Check sheet for the modelled part. Datum: model origin and axes. Units: mm. Face numbers are marked on the shaded views. A direction names the side the tool comes from. Give positions to 0.01 mm unless a question says otherwise; leave off trailing zeros. Order: outer loops, then holes, each group sorted by start corner. A loop starts at its lowest first (then second) coordinate and runs counter-clockwise, first axis right, second up.
from build123d import *

# Parameters (mm, degrees)
ESQUISSE1_R             = 6
BOSS_EXTRU_1_DEPTH      = 100
ESQUISSE2_R             = 6
BOSS_EXTRU_2_DEPTH      = 5
BOSS_EXTRU_3_START      = 5
ESQUISSE3_R             = 6
BOSS_EXTRU_3_DEPTH      = 5
ENL_V_MAT_EXTRU_1_DEPTH = 20
ENL_V_MAT_EXTRU_3_REACH = 126.126
ESQUISSE5_W             = 72.5
ESQUISSE5_H             = 20
ESQUISSE6_W             = 72.5
ESQUISSE6_H             = 6
ENL_V_MAT_EXTRU_4_DEPTH = 40
ENL_V_MAT_EXTRU_5_DEPTH = 10
ENL_V_MAT_EXTRU_6_DEPTH = 10


with BuildPart() as part:
    # Esquisse1 → Boss.-Extru.1 (new body)
    with BuildSketch(Plane(origin=(0, 0, 0), x_dir=(0, 0, -1), z_dir=(1, 0, 0))):
        with BuildLine():
            Line((48.5526258, 0), (0, 0))
            Line((0, 0), (0, 15))
            Line((0, 15), (15, 15))
            Line((15, 15), (15, 19))
            ThreePointArc((15, 19), (9, 25), (15, 31))
            Line((15, 31), (15, 35))
            Line((15, 35), (-15, 35))
            Line((-15, 35), (-36.4473742, 15))
            Line((-36.4473742, 15), (-36.4473742, -10))
            Line((-36.4473742, -10), (48.5526258, -10))
            Line((48.5526258, -10), (48.5526258, 0))
        make_face()
        with Locations((15, 25)):
            Circle(ESQUISSE1_R)
    extrude(amount=BOSS_EXTRU_1_DEPTH)

    # Esquisse2 → Boss.-Extru.2 (add)
    with BuildSketch(Plane(origin=(100, 0, 0), x_dir=(0, 0, -1), z_dir=(1, 0, 0))):
        with Locations(Location((15, 25, 0), (0, 0, 90))):
            Circle(ESQUISSE2_R)
    extrude(amount=BOSS_EXTRU_2_DEPTH)

    # Esquisse3 → Boss.-Extru.3 (add)
    with BuildSketch(Plane.ZY.offset(BOSS_EXTRU_3_START)):
        with Locations((-15, 25)):
            Circle(ESQUISSE3_R)
    extrude(amount=-BOSS_EXTRU_3_DEPTH)

    # Esquisse4 → Enlèv. mat.-Extru.1 (cut)
    with BuildSketch(Plane(origin=(0, 26.202468667, 24.434197326), x_dir=(1, 0, 0), z_dir=(0, 0.7313537016191716, 0.6819983600624975))):
        with BuildLine():
            ThreePointArc((107.5, -1.763154778), (105.303300859, 3.54014608), (100, 5.736845222))
            Line((100, 5.736845222), (100, -1.763154778))
            Line((100, -1.763154778), (100, -9.263154778))
            ThreePointArc((100, -9.263154778), (105.303300859, -7.066455637), (107.5, -1.763154778))
        make_face()
        with BuildLine():
            Line((100, -1.763154778), (100, 5.736845222))
            ThreePointArc((100, 5.736845222), (92.5, -1.763154778), (100, -9.263154778))
            Line((100, -9.263154778), (100, -1.763154778))
        make_face()
    extrude(amount=-ENL_V_MAT_EXTRU_1_DEPTH, mode=Mode.SUBTRACT)

    # Enlèv. mat.-Extru.3: up to this face of the body (flat: up to its plane)
    enl_v_mat_extru_3_end = Plane(part.part.faces().sort_by_distance((50, 0, -24.2763129))[0])
    # Esquisse5 → Enlèv. mat.-Extru.3 (cut, up to the picked face)
    with BuildSketch(Plane(origin=(0, 35, 0), x_dir=(1, 0, 0), z_dir=(0, 1, 0)), mode=Mode.PRIVATE) as enl_v_mat_extru_3_sk1:
        with Locations((46.25, 5)):
            Rectangle(ESQUISSE5_W, ESQUISSE5_H)
    enl_v_mat_extru_3_tool1 = split(extrude(enl_v_mat_extru_3_sk1.sketch, amount=-ENL_V_MAT_EXTRU_3_REACH, mode=Mode.PRIVATE), bisect_by=enl_v_mat_extru_3_end, keep=Keep.BOTH, mode=Mode.PRIVATE)
    add(enl_v_mat_extru_3_tool1.solids().sort_by(Axis((46.25, 35, -5), (0, -1, 0)))[0], mode=Mode.SUBTRACT)

    # Esquisse6 → Enlèv. mat.-Extru.4 (cut)
    with BuildSketch(Plane(origin=(0, 0, 0), x_dir=(1, 0, 0), z_dir=(0, 1, 0))):
        with Locations((46.25, 18)):
            Rectangle(ESQUISSE6_W, ESQUISSE6_H)
    extrude(amount=ENL_V_MAT_EXTRU_4_DEPTH, mode=Mode.SUBTRACT)

    # Esquisse7 → Enlèv. mat.-Extru.5 (cut)
    with BuildSketch(Plane.XZ.offset(10)):
        with BuildLine():
            ThreePointArc((22.5, -8.148997132), (15, -0.648997132), (7.5, -8.148997132))
            Line((7.5, -8.148997132), (15, -8.148997132))
            Line((15, -8.148997132), (22.5, -8.148997132))
        make_face()
        with BuildLine():
            Line((15, -8.148997132), (7.5, -8.148997132))
            ThreePointArc((7.5, -8.148997132), (15, -15.648997132), (22.5, -8.148997132))
            Line((22.5, -8.148997132), (15, -8.148997132))
        make_face()
        with BuildLine():
            ThreePointArc((35, -0.648997132), (29.696699141, -2.845696273), (27.5, -8.148997132))
            Line((27.5, -8.148997132), (35, -8.148997132))
            Line((35, -8.148997132), (65, -8.148997132))
            Line((65, -8.148997132), (72.5, -8.148997132))
            ThreePointArc((72.5, -8.148997132), (70.303300859, -2.845696273), (65, -0.648997132))
            Line((65, -0.648997132), (35, -0.648997132))
        make_face()
        with BuildLine():
            Line((35, -8.148997132), (27.5, -8.148997132))
            ThreePointArc((27.5, -8.148997132), (29.696699141, -13.452297991), (35, -15.648997132))
            Line((35, -15.648997132), (65, -15.648997132))
            ThreePointArc((65, -15.648997132), (70.303300859, -13.452297991), (72.5, -8.148997132))
            Line((72.5, -8.148997132), (65, -8.148997132))
            Line((65, -8.148997132), (35, -8.148997132))
        make_face()
        with BuildLine():
            ThreePointArc((92.5, -8.148997132), (85, -0.648997132), (77.5, -8.148997132))
            Line((77.5, -8.148997132), (85, -8.148997132))
            Line((85, -8.148997132), (92.5, -8.148997132))
        make_face()
        with BuildLine():
            Line((85, -8.148997132), (77.5, -8.148997132))
            ThreePointArc((77.5, -8.148997132), (85, -15.648997132), (92.5, -8.148997132))
            Line((92.5, -8.148997132), (85, -8.148997132))
        make_face()
    extrude(amount=-ENL_V_MAT_EXTRU_5_DEPTH, mode=Mode.SUBTRACT)

    # Esquisse8 → Enlèv. mat.-Extru.6 (cut)
    with BuildSketch(Plane.XZ.offset(10)):
        Polygon((100, -48.5526258), (100, -38.5526258), (90, -48.5526258), align=None)
    extrude(amount=-ENL_V_MAT_EXTRU_6_DEPTH, mode=Mode.SUBTRACT)


solid = part.part
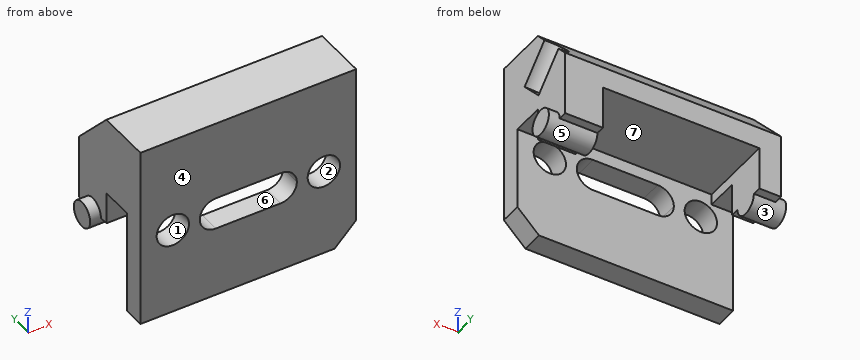
1) Section check B-B, the plane y = -4.5. Record the cut outline in (x, z).
Recorded:
outline: (0, -48.55) - (90, -48.55) - (100, -38.55) - (100, 36.45) - (0, 36.45) - close; hole circle Ø15 at (15, -8.15); hole (35, -15.65) - (65, -15.65) arc R7.5 ccw to (65, -0.65) - (35, -0.65) arc R7.5 ccw to start; hole circle Ø15 at (85, -8.15)
2) Draft check along Z on the marked faces 1, 2, 3 and 4. Enter one of: +Z half, -Z half, draft (parallel to the pull), parting line (faces both ways), or undercut.
Recorded:
face 1: undercut
face 2: undercut
face 3: parting line
face 4: draft
3) Material ranges on L1, parallel to Z at x = 85, y = -3; L2, parallel to X at y = -8, z = -3; L3, parallel to X at y = 32, z = -9, recorded low to high.
Recorded:
L1: z = -48.55 to -15.65, -0.65 to 36.45
L2: x = 0 to 9.55, 20.45 to 29.55, 70.45 to 79.55, 90.45 to 100
L3: x = 0 to 10, 82.5 to 100
4) Depth check by flat-ended pin: pin 1 Ø6 at (x, y) = (29, 20.5) entering from -Z; pin 2 Ø8 at (x, z) = (58, -11.5) entering from +Y; pin 3 Ø3 at (x, y) = (87.5, 24) entering from -Z; pin 4 Ø4 at (x, y) = (88, 2.5) entering from -Z. Enter the tip coordinate at first touch or a pass-through.
Recorded:
pin 1: stops at z = 5
pin 2: passes through
pin 3: stops at z = -21
pin 4: stops at z = 0
5) Section check C-C, the plane x = 74.5. Record the cut outline in (y, z).
Recorded:
outline: (-10, -48.55) - (0, -48.55) - (0, 5) - (35, 5) - (35, 15) - (15, 36.45) - (-10, 36.45) - close
6) Section check D-D, the plane z = -37. Record the cut outline in (x, y).
Recorded:
outline: (0, -10) - (100, -10) - (100, 0) - (0, 0) - close
7) Section check A-A, the plane x = 15. Record the cut outline in (y, z).
Recorded:
outline: (-10, -48.55) - (0, -48.55) - (0, -15.65) - (-10, -15.65) - close; (-10, -0.65) - (0, -0.65) - (0, 5) - (35, 5) - (35, 15) - (15, 36.45) - (-10, 36.45) - close
8) Set-up check for the marked faces 5, 6 and 7: record each of +Z, -Z, +X, -X, +Y, -Y from which the full face is reachable in a straight line by a thin tool's end or side.
Recorded:
face 5: +X
face 6: +Y, -Y
face 7: -Z, +Y
